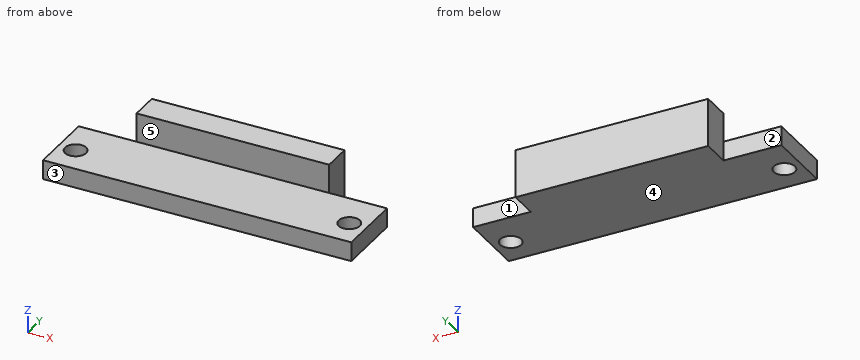
from build123d import *

# Parameters (mm, degrees)
SKETCH_1_W          = 32
SKETCH_1_H          = 7
EXTRUDE_1_DEPTH     = 2
SKETCH_2_R          = 1.1
CUT_EXTRUDE_1_DEPTH = 2
SKETCH_3_W          = 20
SKETCH_3_H          = 3
EXTRUDE_2_DEPTH     = 5


with BuildPart() as part:
    # 草图1 → 凸台-拉伸1 (new body)
    with BuildSketch(Plane.XY):
        with Locations((16, 3.5)):
            Rectangle(SKETCH_1_W, SKETCH_1_H)
    extrude(amount=EXTRUDE_1_DEPTH)

    # 草图2 → 切除-拉伸1 (cut)
    with BuildSketch(Plane(origin=(0, 0, 0), x_dir=(-1, 0, 0), z_dir=(0, 0, -1))):
        with Locations((-30.2, 3)):
            Circle(SKETCH_2_R)
        with Locations((-1.8, 3)):
            Circle(SKETCH_2_R)
    extrude(amount=-CUT_EXTRUDE_1_DEPTH, mode=Mode.SUBTRACT)

    # 草图3 → 凸台-拉伸2 (add)
    with BuildSketch(Plane(origin=(0, 0, 0), x_dir=(-1, 0, 0), z_dir=(0, 0, -1))):
        with Locations((-16, 8.5)):
            Rectangle(SKETCH_3_W, SKETCH_3_H)
    extrude(amount=-EXTRUDE_2_DEPTH)


solid = part.part
Design review of the part built by this model. Coordinates are the model's own, in mm. Face numbers are marked on the shaded views. A direction names the side the tool comes from. Coordinates: 2 decimals unless noted, no trailing zeros. Order: outer loops, then holes, each group sorted by start corner. A loop starts at its lowest first (then second) coordinate and runs counter-clockwise, first axis right, second up. Notation, with made-up numbers: (19.5, 79.5) -> (62.5, 79.5) arc R25 ccw to (62.5, 97.5) -> close; hole circle Ø9 at (12, -38). An arc over 180 degrees is marked (long way). Use one line per item in the form item = value. Start each with the question number.
(1) Add section B-B on x = 1.8. State the section outline as (y, z) points.
(2) Add section D-D on y = 7.75. State the section outline as (x, z) points.
(3) Add section A-A on y = 3. State the section outline as (x, z) points, plus the area to 3 significant figures.
(4) Add section C-C on x = 10.5. State the section outline as (y, z) points, plus the area to 3 significant figures.
(5) For probe 1 along Y at (x, z) = (1.8, 0.9); probe 2 along X at (y, z) = (8, 2.5); probe 3 along Z at (x, y) = (2, 1), list the stretches that pass through material, from the lowest coordinate up.
(6) For the marked faces 1, 2, 3, 4 and 5, list the 3-axis set-ups (+Z, -Z, +X, -X, +Y, -Y) from which the entire face can be reached by the end or side of a thin tool; tool diameter is ignored.
(7) Insertion check: pin 1 (1.8 mm diameter, centred on x = 1.8, y = 3, fed in from -Z); pin 2 (1.5 mm diameter, centred on y = 8, z = 3, fed in from +X); pin 3 (3.5 mm diameter, centred on x = 9, y = 5, fed in from +Z); pin 4 (2 mm diameter, centred on x = 28.5, z = 0.5, fed in from +Y). Each pin has a flat end and moves straight along its axis. Give the tip position at first contact, or say it passes through.
Answer block:
q1.outline = (0, 0) -> (1.9, 0) -> (1.9, 2) -> (0, 2) -> close; (4.1, 0) -> (7, 0) -> (7, 2) -> (4.1, 2) -> close
q2.outline = (6, 0) -> (26, 0) -> (26, 5) -> (6, 5) -> close
q3.outline = (0, 0) -> (0.7, 0) -> (0.7, 2) -> (0, 2) -> close; (2.9, 0) -> (29.1, 0) -> (29.1, 2) -> (2.9, 2) -> close; (31.3, 0) -> (32, 0) -> (32, 2) -> (31.3, 2) -> close
q3.area = 55.2 mm²
q4.outline = (0, 0) -> (10, 0) -> (10, 5) -> (7, 5) -> (7, 2) -> (0, 2) -> close
q4.area = 29.0 mm²
q5.probe_1 = 0 to 1.9, 4.1 to 7
q5.probe_2 = 6 to 26
q5.probe_3 = 0 to 2
q6.face_1 = +Z, -Z, +X, +Y
q6.face_2 = +Z, -Z, -X, +Y
q6.face_3 = +Z, -Z, +X, -X, -Y
q6.face_4 = -Z, +X, -X, +Y, -Y
q6.face_5 = +Z, +X, -X, -Y
q7.pin_1 = through
q7.pin_2 = 26
q7.pin_3 = 2
q7.pin_4 = 7
